```python
from build123d import *

# Parameters (mm, degrees)
F0_W      = 25.2578889922
F0_H      = 87.7920170172
F0_W_2    = 241.5705997671
F0_H_2    = 156.5749233454
F0_W_3    = 60
F0_H_3    = 200
F4_DEPTH  = 75
F3_R      = 12.5698897047
F5_DEPTH  = 5000
F6_W      = 180
F6_H      = 130
F7_DEPTH  = 6000
F8_R      = 30
F8_R_2    = 25
F9_DEPTH  = 75
F11_W     = 40000
F11_H     = 33
F12_DEPTH = 15000
F13_DEPTH = 1000
F14_DEPTH = 1000
F15_DEPTH = 350
F16_R     = 15


with BuildPart() as f1:
    # F0 (on Top) → F1 (revolve)
    with BuildSketch(Plane.XY):
        with Locations((58.379718929, 43.8960085086)):
            Rectangle(F0_W, F0_H)
    revolve(axis=Axis((58.379718929, 0, 0), (1, 0, 0)))


with BuildPart() as f2:
    # F0 (on Top) → F2 (revolve)
    with BuildSketch(Plane.XY):
        with Locations((218.8274469054, 78.2874616727)):
            Rectangle(F0_W_2, F0_H_2)
    revolve(axis=Axis((218.8274469054, 0, 0), (1, 0, 0)))


with BuildPart() as f4:
    # F0 (on Top) → F4 (new body, symmetric)
    with BuildSketch(Plane.XY):
        Rectangle(F0_W_3, F0_H_3)
    extrude(amount=F4_DEPTH, both=True)


with BuildPart() as f5_tool:
    # F3 (on Right) → F5 (new body, symmetric)
    with BuildSketch(Plane.YZ):
        Circle(F3_R)
    extrude(amount=F5_DEPTH, both=True)


with BuildPart() as f1_1:
    add(f1.part)

    # F5: cut by f5_tool
    add(f5_tool.part, mode=Mode.SUBTRACT)



with BuildPart() as f2_1:
    add(f2.part)

    # F5: cut by f5_tool
    add(f5_tool.part, mode=Mode.SUBTRACT)


with BuildPart() as f4_1:
    add(f4.part)

    # F5: cut by f5_tool
    add(f5_tool.part, mode=Mode.SUBTRACT)

    # F6 (on Right) → F7 (cut)
    with BuildSketch(Plane.YZ):
        Rectangle(F6_W, F6_H)
    extrude(amount=-F7_DEPTH, mode=Mode.SUBTRACT)

    # F8 (on Top) → F9 (join, symmetric)
    with BuildSketch(Plane.XY):
        with Locations((-30, 90)):
            Circle(F8_R)
        with Locations((-30, 90)):
            Circle(F8_R_2, mode=Mode.SUBTRACT)
        with Locations((-30, -90)):
            Circle(F8_R)
        with Locations((-30, -90)):
            Circle(F8_R_2, mode=Mode.SUBTRACT)
    extrude(amount=F9_DEPTH, both=True)

    # F11 (on offset) → F12 (cut)
    with BuildSketch(Plane.YZ.offset(-10)):
        Rectangle(F11_W, F11_H)
    extrude(amount=-F12_DEPTH, mode=Mode.SUBTRACT)

    # F8 (on Top) → F13 (cut, symmetric)
    with BuildSketch(Plane.XY):
        with Locations((-30, 90)):
            Circle(F8_R_2)
    extrude(amount=F13_DEPTH, both=True, mode=Mode.SUBTRACT)

    # F8 (on Top) → F14 (cut, symmetric)
    with BuildSketch(Plane.XY):
        with Locations((-30, -90)):
            Circle(F8_R_2)
    extrude(amount=F14_DEPTH, both=True, mode=Mode.SUBTRACT)


with BuildPart() as f1_2:
    add(f1_1.part)

    add(f2_1.part)  # F15 merges F2

    add(f4_1.part)  # F15 merges F4
    # F3 (on Right) → F15 (join)
    with BuildSketch(Plane.YZ):
        Circle(F3_R)
    extrude(amount=F15_DEPTH)

    # F16
    f16_edges = [f1_2.edges().sort_by_distance(p)[0] for p in [
        (339.612747, -156.574923, 0),
        (98.042147, -156.574923, 0),
    ]]
    fillet(f16_edges, radius=F16_R)


solid = f1_2.part
```
Build history of the part. All positions in model axes, mm. A direction names the side the tool comes from. Coordinates: 2 decimals unless noted, no trailing zeros. Order: outer loops, then holes, each group sorted by start corner. A loop starts at its lowest first (then second) coordinate and runs counter-clockwise, first axis right, second up.
Item 1: Drop flat-ended pins along their axis: pin 1 Ø6 at (x, z) = (184, -99) entering from +Y; pin 2 Ø3 at (x, y) = (281, -76) entering from +Z; pin 3 Ø12 at (x, z) = (176.5, 122.5) entering from +Y. Give the stop position or say it passes through.
Filled in:
pin 1: stops at y = 123.69
pin 2: stops at z = 137.72
pin 3: stops at y = 104.61
Item 2: Drill centre lines: L1, parallel to Y at x = -30, z = 36; L2, parallel to X at y = 14, z = 71.5; L3, parallel to X at y = -53, z = -27.5. Where is each one in solid material? Low to high.
Filled in:
L1: y = -120 to -115, -65 to -60, 60 to 65, 115 to 120
L2: x = -30 to 30, 45.75 to 71.01, 98.04 to 339.61
L3: x = 0 to 30, 45.75 to 71.01, 98.04 to 339.61
Item 3: Mould opens along X. For faces 5 (the cylindrical face through (-7.28, -109.59, 1.05)), 6 (the cylindrical face through (344.734, -2.725, -12.271)), 7 (the flat face through (350, 0, 0)) say: released by +X, released by -X, zero draft, split by the parting line, or undercut.
Filled in:
face 5: undercut
face 6: zero draft
face 7: released by +X
Item 4: Saw through at C-C on y = -80. State how many separate pieces and enclosed holes the cut face has, then the cut area to 3 significant figures.
Filled in:
separate pieces: 5
enclosed holes: 1
area: 72,600 mm2
Item 5: Tool access for faces 1 (the flat face through (-30, -1, -70)), 2 (the cylindrical face through (58.56, 83.74, 26.37)), 3 (the flat face through (-6, 2, 75)), 4 (the flat face through (-55.3, 89.9, -16.5)): list every direction of +Z, -Z, +X, -X, +Y, -Y with a clear straight run to the whole face (end or side of a thin tool).
Filled in:
face 1: +Z, -Z, -X
face 2: none
face 3: +Z, -X, +Y, -Y
face 4: -X, +Y, -Y
Item 6: Saw through at B-B on x = 159.5. List the corners of the cut face in (y, z).
Filled in:
outline: circle Ø313.15 at (0, 0)
